Geometry check sheet. Reference: drawing and pictorial views, mm from the part's lowest x, y, z. A direction names the side the tool comes from. Round coordinates to 2 decimals unless told otherwise and drop trailing zeros. Order: outer loops, then holes, each group sorted by start corner. A loop starts at its lowest first (then second) coordinate and runs counter-clockwise, first axis right, second up.
(1) Thickness scan on L1, parallel to X at y = 2.1, z = 3.5; L2, parallel to X at y = 0.55, z = 1; L3, parallel to Y at x = 6.75, z = 10.75. Record the ranges inside material, lowest first.
(2) Cross-section at B-B on x = 10.25. Enter the section's corners in (y, z), and give its area (3 significant figures).
(3) Cross-section at A-A on y = 2. Enter the section's corners in (x, z), and give its area (3 significant figures).
(4) Gauge pin test, flat ends, axial feed: P1, Ø1, axis at y = 3.5, z = 3, coming from the +X side; P2, Ø1.5, axis at x = 9.5, z = 1.5, coming from the -Y side; P3, Ø2, axis at x = 5, z = 10, coming from the +Y side. Record the tip position at first contact, or that the pin passes through.
(5) Set-up check for the marked faces 1, 2, 3 and 4: record each of +Z, -Z, +X, -X, +Y, -Y from which the full face is reachable in a straight line by a thin tool's end or side.
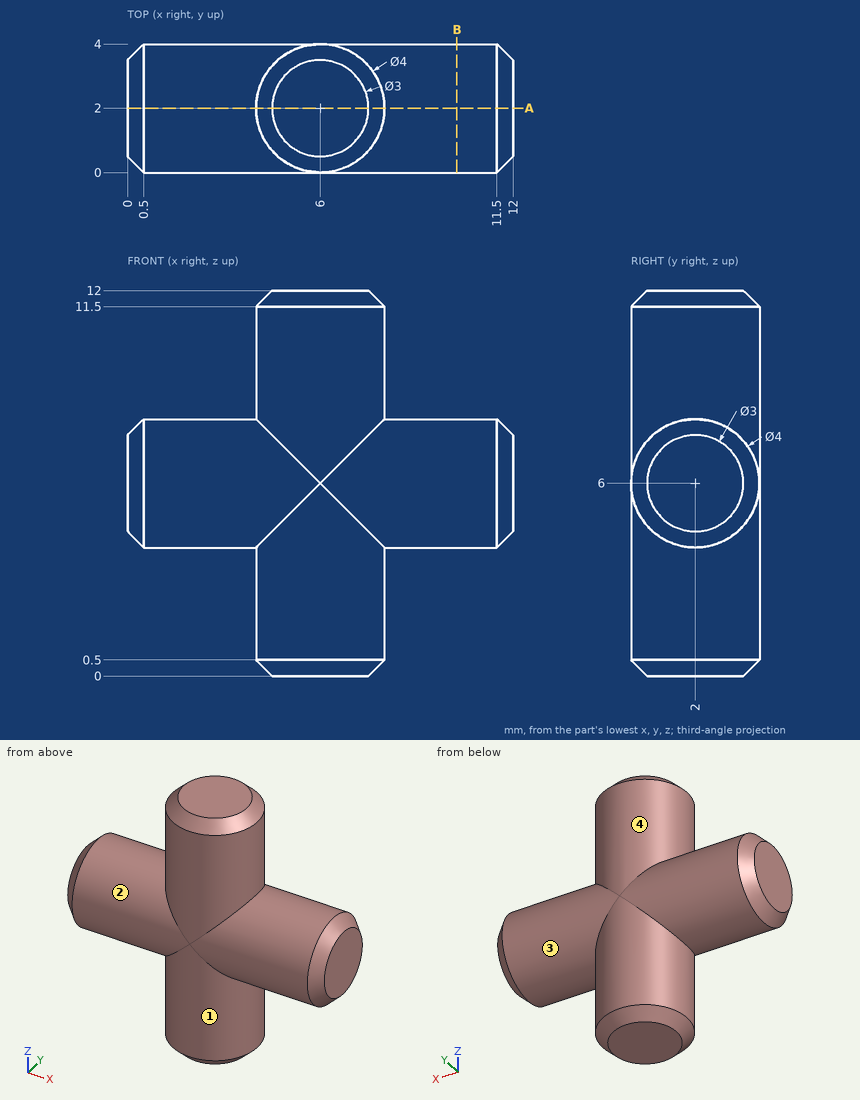
Found:
1. L1: x = 4 to 8
1. L2: x = 4.62 to 7.38
1. L3: y = 0.15 to 3.85
2. outline: circle Ø4 at (2, 6)
2. area: 12.6 mm2
3. outline: (0, 4.5) - (0.5, 4) - (4, 4) - (4, 0.5) - (4.5, 0) - (7.5, 0) - (8, 0.5) - (8, 4) - (11.5, 4) - (12, 4.5) - (12, 7.5) - (11.5, 8) - (8, 8) - (8, 11.5) - (7.5, 12) - (4.5, 12) - (4, 11.5) - (4, 8) - (0.5, 8) - (0, 7.5) - close
3. area: 79.0 mm2
4. P1: stops at x = 7.73
4. P2: passes through
4. P3: stops at y = 4
5. face 1: -Z
5. face 2: -X
5. face 3: +X
5. face 4: +Z
